from build123d import *

# Parameters (mm, degrees)
SKETCH_1_R          = 2.6
SKETCH_1_W          = 2
SKETCH_1_H          = 13.6
EXTRUDE_1_DEPTH     = 2
SKETCH_1_3_W        = 1.5
SKETCH_1_3_H        = 13.6
SKETCH_1_3_W_2      = 2
EXTRUDE_2_DEPTH     = 1.8
SKETCH_1_5_R        = 2.6
CUT_EXTRUDE_1_DEPTH = 1
FILLET_1_R          = 2
FILLET_2_R          = 1.5
FILLET_3_R          = 1.2


with BuildPart() as part:
    # Sketch 1 → Extrude 1 (new body)
    with BuildSketch(Plane(origin=(0, 0, 0), x_dir=(1, 0, 0), z_dir=(0, 1, 0))):
        Polygon((34.55, 18.6), (-34.55, 18.6), (-34.55, -18.6), (34.55, -18.6), (34.55, -6.8), (32.55, -6.8), (32.55, 6.8), (34.55, 6.8), align=None)
        with Locations((-29.75, -7.1)):
            Circle(SKETCH_1_R, mode=Mode.SUBTRACT)
        with Locations((-29.75, 7.1)):
            Circle(SKETCH_1_R, mode=Mode.SUBTRACT)
        with Locations((33.55, 0)):
            Rectangle(SKETCH_1_W, SKETCH_1_H)
        with Locations((-29.75, -7.1)):
            Circle(SKETCH_1_R)
        with Locations((-29.75, 7.1)):
            Circle(SKETCH_1_R)
    extrude(amount=EXTRUDE_1_DEPTH)

    # Sketch 1_3 → Extrude 2 (add)
    with BuildSketch(Plane(origin=(0, 0, 0), x_dir=(1, 0, 0), z_dir=(0, 1, 0))):
        with Locations((35.3, 0)):
            Rectangle(SKETCH_1_3_W, SKETCH_1_3_H)
        with Locations((33.55, 0)):
            Rectangle(SKETCH_1_3_W_2, SKETCH_1_3_H)
    extrude(amount=-EXTRUDE_2_DEPTH)

    # Sketch 1_5 → Cut-Extrude 1 (cut)
    with BuildSketch(Plane(origin=(0, 0, 0), x_dir=(1, 0, 0), z_dir=(0, 1, 0))):
        with Locations((-29.75, -7.1)):
            Circle(SKETCH_1_5_R)
        with Locations((-29.75, 7.1)):
            Circle(SKETCH_1_5_R)
    extrude(amount=CUT_EXTRUDE_1_DEPTH, mode=Mode.SUBTRACT)

    # Fillet 1
    fillet_1_edges = [part.edges().sort_by_distance(p)[0] for p in [
        (-34.55, 1, 18.6),
        (-34.55, 1, -18.6),
        (34.55, 1, -18.6),
        (34.55, 1, 18.6),
    ]]
    fillet(fillet_1_edges, radius=FILLET_1_R)

    # Fillet 2
    fillet_2_edges = [part.edges().sort_by_distance(p)[0] for p in [
        (36.05, -0.9, -6.8),
        (36.05, -0.9, 6.8),
    ]]
    fillet(fillet_2_edges, radius=FILLET_2_R)

    # Fillet 3
    fillet_3_edges = [part.edges().sort_by_distance(p)[0] for p in [
        (32.55, -1.8, 0),
    ]]
    fillet(fillet_3_edges, radius=FILLET_3_R)


solid = part.part
Input: part model. Units: mm. Frame: model coordinates. A direction names the side the tool comes from. Give positions to 0.01 mm unless a question says otherwise; leave off trailing zeros. Write each loop counter-clockwise with the first axis right and the second up, starting at its lowest first coordinate (ties: lowest second). Pieces come first, ordered by that corner, then holes.
Q1. Section A-A, the plane z = -1. Output: boundary loops of the cut face in (x, y), plus the area to 3 significant figures.
Q2. Pull-direction query (Z, two-part tool) for faces 6 (the face through (-30, 1, 7)), 7 (the face through (-32.347, 0.493, -7.214)), 8 (the face through (34, -1, 6.8)), 9 (the face through (-33.95, 1.01, -18.03)); classes: pulls with the +Z half, pulls with the -Z half, needs draft (parallel to the pull), parting line crosses it, or undercut.
Q3. Section B-B, the plane x = -29.75. Output: boundary loops of the cut face in (y, z), plus the area to 3 significant figures.
Q4. First-contact query: P1, Ø18.5, axis at x = 14.5, z = -3.5, coming from the -Y side; P2, Ø1.2, axis at x = 35.5, z = 3, coming from the +Y side; P3, Ø0.5, axis at x = 33.5, y = -0.5, coming from the -Z side. Flat tips, straight axial feed; report the tip coordinate or a pass-through.
Q5. Material intervals for probe 1 along Z at (x, y) = (-29.75, 0.45); probe 2 along X at (y, z) = (0.3, -7.1); probe 3 along Y at (x, z) = (30, -2.5), sorted ascending.
Q6. Section C-C, the plane z = 14.5. Output: boundary loops of the cut face in (x, y).
Q7. Section D-D, the plane x = -8. Output: boundary loops of the cut face in (y, z).
Q8. Set-up query: faces 1 (the face through (-32.347, 0.493, 6.986)), 2 (the face through (0, 1, -18.6)), 3 (the face through (34, -1, -6.8)), 4 (the face through (34.55, 1, 0)), 5 (the face through (-34.55, 1, 0)). Return all of +Z, -Z, +X, -X, +Y, -Y with unobstructed straight access to the full face (end or side cutting, diameter ignored); none if empty.
Filled in:
1. outline: (-34.55, 0) - (32.55, 0) - (32.55, -0.6) arc R1.2 ccw to (33.75, -1.8) - (36.05, -1.8) - (36.05, 0) - (34.55, 0) - (34.55, 2) - (-34.55, 2) - close
1. area: 144 mm2
2. face 6: undercut
2. face 7: undercut
2. face 8: pulls with the +Z half
2. face 9: pulls with the -Z half
3. outline: (0, -18.6) - (2, -18.6) - (2, 18.6) - (0, 18.6) - (0, 9.7) - (1, 9.7) - (1, 4.5) - (0, 4.5) - (0, -4.5) - (1, -4.5) - (1, -9.7) - (0, -9.7) - close
3. area: 64.0 mm2
4. P1: stops at y = 0
4. P2: stops at y = 0
4. P3: stops at z = -6.8
5. probe 1: z = -18.6 to -9.7, -4.5 to 4.5, 9.7 to 18.6
5. probe 2: x = -34.55 to -32.35, -27.15 to 34.55
5. probe 3: y = 0 to 2
6. outline: (-34.55, 0) - (34.55, 0) - (34.55, 2) - (-34.55, 2) - close
7. outline: (0, -18.6) - (2, -18.6) - (2, 18.6) - (0, 18.6) - close
8. face 1: -Y
8. face 2: -Z, +X, -X, +Y, -Y
8. face 3: -Z, +X, -X, -Y
8. face 4: +Z, -Z, +X, +Y
8. face 5: +Z, -Z, -X, +Y, -Y
